Read the model definition and answer for the solid it produces. Units are mm, in the model's axes. Coordinates: 2 decimals unless noted, no trailing zeros. Loops run counter-clockwise (first coordinate to the right, second up) from the corner with the lowest first, then second, coordinate; pieces in that order, holes last.
Q1. Section C-C (x = 0) is taken. Give the vertices of the cut face in (y, z).
Q2. Section A-A (y = 7) is taken. Give the vertices of the cut face in (x, z).
Q3. Flat-ended cylindrical pins translate along their axes: P1, Ø1, axis at x = 1.5, z = -21.5, coming from the +Y side; P2, Ø1.5, axis at x = -1, z = -9.5, coming from the +Y side. Find the tip coordinate at first contact, or state that the pin passes through.
Q4. Section D-D (z = -30) is taken. Give the vertices of the cut face in (x, y), then the cut area to 3 significant figures.
Q5. Section B-B (z = 26.5) is taken. Give the vertices of the cut face in (x, y), then the cut area to 3 significant figures.
Q6. Straight lines are drawn through the part: line 1 (Z direction, x = -0.25, y = 0.75); line 2 (Z direction, x = 0, y = 0.8); line 3 (X direction, y = 9, z = -11). For each, find the intervals that lie inside material, in ascending order.
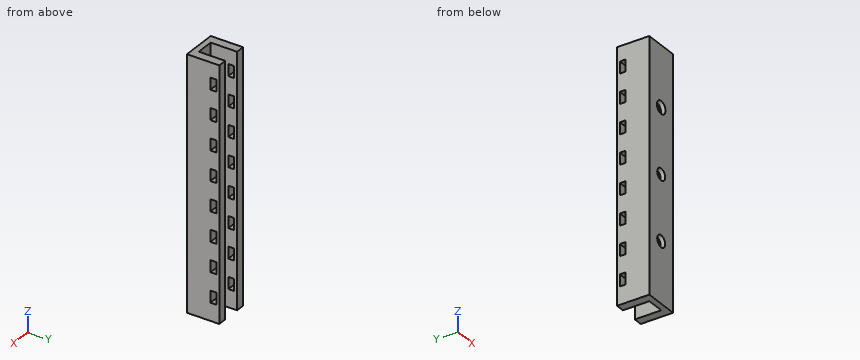
Autodesk Inventor part; units mm, degrees
ref_plane "YZ Plane" through (0, 0, 0) normal (1, 0, 0) x (0, 1, 0)
ref_plane "XZ Plane" through (0, 0, 0) normal (0, 1, 0) x (-1, 0, 0)
ref_plane "XY Plane" through (0, 0, 0) normal (0, 0, 1) x (1, 0, 0)
sketch "Эскиз1" plane through (0, 0, 0) normal (0, 1, 0) x (-1, 0, 0)
  line L0 (-6, -42.5) -> (6, -42.5)
  line L1 (6, -42.5) -> (6, 42.5)
  line L2 (6, 42.5) -> (-6, 42.5)
  line L3 (-6, 42.5) -> (-6, -42.5)
  line L4 (-6, -42.5) -> (6, 42.5) construction
  line L5 (6, -42.5) -> (-6, 42.5) construction
  circle A0 centre (0, 0) radius 2
  circle A1 centre (0, 22) radius 2.1514
  circle A2 centre (0, -22) radius 2
  dimension "d0" = 4
  dimension "d1" = 22
  dimension "d2" = 22
  dimension "d3" = 85
  dimension "d4" = 12
extrude "Выдавливание1" add sketch "Эскиз1" along normal blind 2
sketch "Эскиз2" plane through (0, 2, 0) normal (0, 1, 0) x (1, 0, 0)
  line L0 (-6, 42.5) -> (-6, -42.5)
  line L1 (-6, -42.5) -> (6, -42.5)
  line L2 (6, -42.5) -> (6, 42.5)
  line L3 (6, 42.5) -> (-6, 42.5)
  circle A0 centre (0, 0) radius 2
  circle A1 centre (0, -22) radius 2.1514
  circle A2 centre (0, 22) radius 2
  line L4 (-6, -42.5) -> (-3, -42.5)
  line L5 (-3, -42.5) -> (-3, 42.5)
  line L6 (-3, 42.5) -> (-6, 42.5)
  line L7 (-6, 42.5) -> (-6, -42.5)
  line L8 (6, 42.5) -> (3, 42.5)
  line L9 (3, 42.5) -> (3, -42.5)
  line L10 (3, -42.5) -> (6, -42.5)
  line L11 (6, -42.5) -> (6, 42.5)
  dimension "d7" = 3
  dimension "d8" = 3
extrude "Выдавливание2" add sketch "Эскиз2" along normal blind 9 contours L3 L5 L1 L0 | L3 L2 L1 L9
chamfer "Фаска1" distance 0.5 angle 45 1 edges at (2.1514, 2, 22)
chamfer "Фаска2" distance 0.5 angle 45 2 edges at (2, 2, 0) (2, 2, -22)
sketch "Эскиз3" plane through (6, 0, 42.5) normal (1, 0, 0) x (0, 0, -1)
  line L0 (5, 10) -> (9, 10)
  line L1 (9, 10) -> (9, 8)
  line L2 (9, 8) -> (5, 8)
  line L3 (5, 8) -> (5, 10)
  line L4 (0, 11) -> (85, 11)
  line L5 (0, 0) -> (0, 11)
  line L6 (15, 10) -> (19, 10)
  line L7 (19, 10) -> (19, 8)
  line L8 (19, 8) -> (15, 8)
  line L9 (15, 8) -> (15, 10)
  line L10 (25, 10) -> (29, 10)
  line L11 (29, 10) -> (29, 8)
  line L12 (29, 8) -> (25, 8)
  line L13 (25, 8) -> (25, 10)
  line L14 (35, 10) -> (39, 10)
  line L15 (39, 10) -> (39, 8)
  line L16 (39, 8) -> (35, 8)
  line L17 (35, 8) -> (35, 10)
  line L18 (45, 10) -> (49, 10)
  line L19 (49, 10) -> (49, 8)
  line L20 (49, 8) -> (45, 8)
  line L21 (45, 8) -> (45, 10)
  line L22 (55, 10) -> (59, 10)
  line L23 (59, 10) -> (59, 8)
  line L24 (59, 8) -> (55, 8)
  line L25 (55, 8) -> (55, 10)
  line L26 (65, 10) -> (69, 10)
  line L27 (69, 10) -> (69, 8)
  line L28 (69, 8) -> (65, 8)
  line L29 (65, 8) -> (65, 10)
  line L30 (75, 10) -> (79, 10)
  line L31 (79, 10) -> (79, 8)
  line L32 (79, 8) -> (75, 8)
  line L33 (75, 8) -> (75, 10)
  point P0 (42.5, 0)
  dimension "d17" = 4
  dimension "d18" = 2
  dimension "d19" = 1
  dimension "d20" = 5
  dimension "d23" = 10
extrude "Выдавливание3" cut sketch "Эскиз3" against normal up to surface (12 mm away)
properties part number "рейка кати"
Numbers:
1. outline: (0, -42.5) - (2, -42.5) - (2, -24.5) - (1.5, -24) - (0, -24) - close; (0, -20) - (1.5, -20) - (2, -19.5) - (2, -2.5) - (1.5, -2) - (0, -2) - close; (0, 2) - (1.5, 2) - (2, 2.5) - (2, 19.35) - (1.5, 19.85) - (0, 19.85) - close; (0, 24.15) - (1.5, 24.15) - (2, 24.65) - (2, 42.5) - (0, 42.5) - close
2. outline: (-6, -42.5) - (-3, -42.5) - (-3, 42.5) - (-6, 42.5) - close; (3, -42.5) - (6, -42.5) - (6, 42.5) - (3, 42.5) - close
3. P1: stops at y = 1.58
3. P2: stops at y = 2
4. outline: (-6, 0) - (6, 0) - (6, 11) - (3, 11) - (3, 2) - (-3, 2) - (-3, 11) - (-6, 11) - close
4. area: 78.0 mm2
5. outline: (-6, 0) - (6, 0) - (6, 8) - (3, 8) - (3, 2) - (-3, 2) - (-3, 8) - (-6, 8) - close; (-6, 10) - (-3, 10) - (-3, 11) - (-6, 11) - close; (3, 10) - (6, 10) - (6, 11) - (3, 11) - close
5. area: 66.0 mm2
6. line 1: z = -42.5 to -23.98, -20.02 to -1.98, 1.98 to 19.86, 24.14 to 42.5
6. line 2: z = -42.5 to -24, -20 to -2, 2 to 19.85, 24.15 to 42.5
6. line 3: x = -6 to -3, 3 to 6
